Verification items for the finished model (mm, model axes). A direction names the side the tool comes from. Give positions to 0.01 mm unless a question says otherwise; leave off trailing zeros. Order: outer loops, then holes, each group sorted by start corner. A loop starts at its lowest first (then second) coordinate and runs counter-clockwise, first axis right, second up. Notation, with made-up numbers: (40.25, 48) - (60.25, 48) arc R21 cw to (60.25, 58) - close; hole circle Ø11 at (69, 79.25). An arc over 180 degrees is marked (long way). Answer as a JSON object with one key per item and string values. Group by question number.
(1) Depth check by flat-ended pin: pin 1 Ø25 at (y, z) = (79.5, 36) entering from +X; pin 2 Ø7 at (x, y) = (-8, 148.5) entering from +Z; pin 3 Ø2 at (x, z) = (182.5, 41) entering from +Y. Enter the tip coordinate at first touch or a pass-through.
(2) Section check D-D (y = 82). Record the boundary of the cut face in (x, z).
(3) Thickness scan on line 1 (Y direction, x = 166.5, z = 27); line 2 (X direction, y = 60, z = 8); line 3 (X direction, y = 94.5, z = 6.5). Record the ranges inside material, lowest first.
(4) Section check C-C (z = 20). Record the boundary of the cut face in (x, y) (3 decimals).
(5) Section check A-A (y = 117). Record the boundary of the cut face in (x, z), then the cut area to 3 significant figures.
(6) Section check B-B (x = 204). Record the boundary of the cut face in (y, z).
(7) Access from +Z, -Z, +X, -X, +Y, -Y to the whole of each face (thin tool, end or side, straight path). Record for faces 4 (the face through (109.733, 54, 24)), 5 (the face through (109.733, 177, 24)), 6 (the face through (-7, 110, 29.464)), 7 (the face through (48, 186.505, 24)).
(8) Mould release check, pull along Y, two halves, no side actions. Record for faces 1 (the face through (48, 189.045, 24)), 2 (the face through (-13.726, 100, 30)), 3 (the face through (108, 100, 0)): +Y half, -Y half, draft (parallel to the pull), parting line (faces both ways), or undercut.
```python
from build123d import *

# Parameters (mm, degrees)
F0_W     = 143.7272205949
F0_H     = 66.6242633015
F1_DEPTH = 49.53
F2_T     = -2.54
F3_W     = 13.7264372474
F3_H     = 19.3594098091
F3_H_2   = 20.8327490836
F3_H_3   = 24.5586633682
F4_DEPTH = 29.464


with BuildPart() as f1:
    # F0 (on Top) → F1 (new body)
    with BuildSketch(Plane.XY):
        Polygon((-16.2664372474, 189.0449970961), (-16.2664372474, 9.442742914), (109.7329184413, 9.442742914), (109.7329184413, 99.243870005), (109.7329184413, 165.8681333065), (109.7329184413, 189.0449970961), align=None)
        with Locations((181.5965287387, 132.5560016558)):
            Rectangle(F0_W, F0_H)
    extrude(amount=F1_DEPTH)

    # F2
    f2_openings = [f1.faces().sort_by_distance(p)[0] for p in [
        (86.832403, 109.148631, 49.53),
        (86.832403, 109.148631, 0),
    ]]
    offset(amount=F2_T, openings=f2_openings, kind=Kind.INTERSECTION)

    # F3 (on Top) → F4 (join)
    with BuildSketch(Plane.XY):
        with Locations((-6.8632186237, 64.5605772734)):
            Rectangle(F3_W, F3_H)
        with Locations((-6.8632186237, 109.6602445468)):
            Rectangle(F3_W, F3_H_2)
        with Locations((-6.8632186237, 153.5996198654)):
            Rectangle(F3_W, F3_H_3)
    extrude(amount=F4_DEPTH)


solid = f1.part
```
Solutions:
{
 "1": {"pin 1": "stops at x = 109.73", "pin 2": "stops at z = 29.46", "pin 3": "stops at y = 165.87"},
 "2": {"outline": "(-16.27, 0) - (-13.73, 0) - (-13.73, 49.53) - (-16.27, 49.53) - close; (107.19, 0) - (109.73, 0) - (109.73, 49.53) - (107.19, 49.53) - close"},
 "3": {"line 1": "y = 99.24 to 101.78, 163.33 to 165.87", "line 2": "x = -16.27 to 0, 107.19 to 109.73", "line 3": "x = -16.27 to -13.73, 107.19 to 109.73"},
 "4": {"outline": "(-16.266, 9.443) - (109.733, 9.443) - (109.733, 99.244) - (253.46, 99.244) - (253.46, 165.868) - (109.733, 165.868) - (109.733, 189.045) - (-16.266, 189.045) - close; hole (-13.726, 11.983) - (107.193, 11.983) - (107.193, 101.784) - (250.92, 101.784) - (250.92, 163.328) - (107.193, 163.328) - (107.193, 186.505) - (-13.726, 186.505) - (-13.726, 165.879) - (0, 165.879) - (0, 141.32) - (-13.726, 141.32) - (-13.726, 120.077) - (0, 120.077) - (0, 99.244) - (-13.726, 99.244) - (-13.726, 74.24) - (0, 74.24) - (0, 54.881) - (-13.726, 54.881) - close"},
 "5": {"outline": "(-16.27, 0) - (0, 0) - (0, 29.46) - (-13.73, 29.46) - (-13.73, 49.53) - (-16.27, 49.53) - close; (250.92, 0) - (253.46, 0) - (253.46, 49.53) - (250.92, 49.53) - close", "area": "656 mm2"},
 "6": {"outline": "(99.24, 0) - (101.78, 0) - (101.78, 49.53) - (99.24, 49.53) - close; (163.33, 0) - (165.87, 0) - (165.87, 49.53) - (163.33, 49.53) - close"},
 "7": {"face 4": "+Z, -Z, +X, -Y", "face 5": "+Z, -Z, +X, +Y", "face 6": "+Z", "face 7": "+Z, -Z"},
 "8": {"face 1": "+Y half", "face 2": "undercut", "face 3": "draft"}
}
